from build123d import *

# Parameters (mm, degrees)
F0_W     = 304.8
F0_H     = 304.8
F1_DEPTH = 25.4
F3_DEPTH = 25.4
F5_DEPTH = 25.4


with BuildPart() as f1:
    # F0 (on Top) → F1 (new body)
    with BuildSketch(Plane.XY):
        Rectangle(F0_W, F0_H)
    extrude(amount=F1_DEPTH)

    # F2 (on face) → F3 (cut)
    with BuildSketch(Plane.XY.offset(25.4)):
        Polygon((152.4, -152.4), (0, 0), (-152.4, -152.4), align=None)
    extrude(amount=-F3_DEPTH, mode=Mode.SUBTRACT)

    # F4 (on face) → F5 (cut)
    with BuildSketch(Plane(origin=(0, 0, 0), x_dir=(1, 0, 0), z_dir=(0, 0, -1))):
        Polygon((2.948233, -152.4), (0, 0), (-152.4, 152.4), (-152.4, -152.4), align=None)
    extrude(amount=-F5_DEPTH, mode=Mode.SUBTRACT)


solid = f1.part
Geometry check sheet. Reference: the model listing, model coordinates, mm. Round coordinates to 2 decimals unless told otherwise and drop trailing zeros. Write each loop counter-clockwise with the first axis right and the second up, starting at its lowest first coordinate (ties: lowest second). Pieces come first, ordered by that corner, then holes. Notation, with made-up numbers: (86, 37.25) - (142, 37.25) arc R33 ccw to (142, 73.25) - close; hole circle Ø8 at (26, 19). An arc over 180 degrees is marked (long way). One line per item, written item: value.
1. Depth check by flat-ended pin: pin 1 Ø5 at (y, z) = (-92.5, 19) entering from -X; pin 2 Ø3 at (x, y) = (86.5, 91) entering from -Z; pin 3 Ø10 at (y, z) = (-61, 7) entering from -X. Enter the tip coordinate at first touch or a pass-through.
The answers:
pin 1: stops at x = 90
pin 2: stops at z = 0
pin 3: stops at x = 56
2. Cross-section at B-B on y = -38. Record the boundary of the cut face in (x, z).
The answers:
outline: (38, 0) - (152.4, 0) - (152.4, 25.4) - (38, 25.4) - close
3. Cross-section at A-A on x = 99.5. Record the boundary of the cut face in (y, z).
The answers:
outline: (-99.5, 0) - (152.4, 0) - (152.4, 25.4) - (-99.5, 25.4) - close
4. Scan lines: L1, parallel to X at y = -61, z = 7; L2, parallel to Y at x = 117.5, z = 10; L3, parallel to X at y = 68.5, z = 2.75. Record each from-to range of solid material in increasing order.
The answers:
L1: x = 61 to 152.4
L2: y = -117.5 to 152.4
L3: x = 1.33 to 152.4
